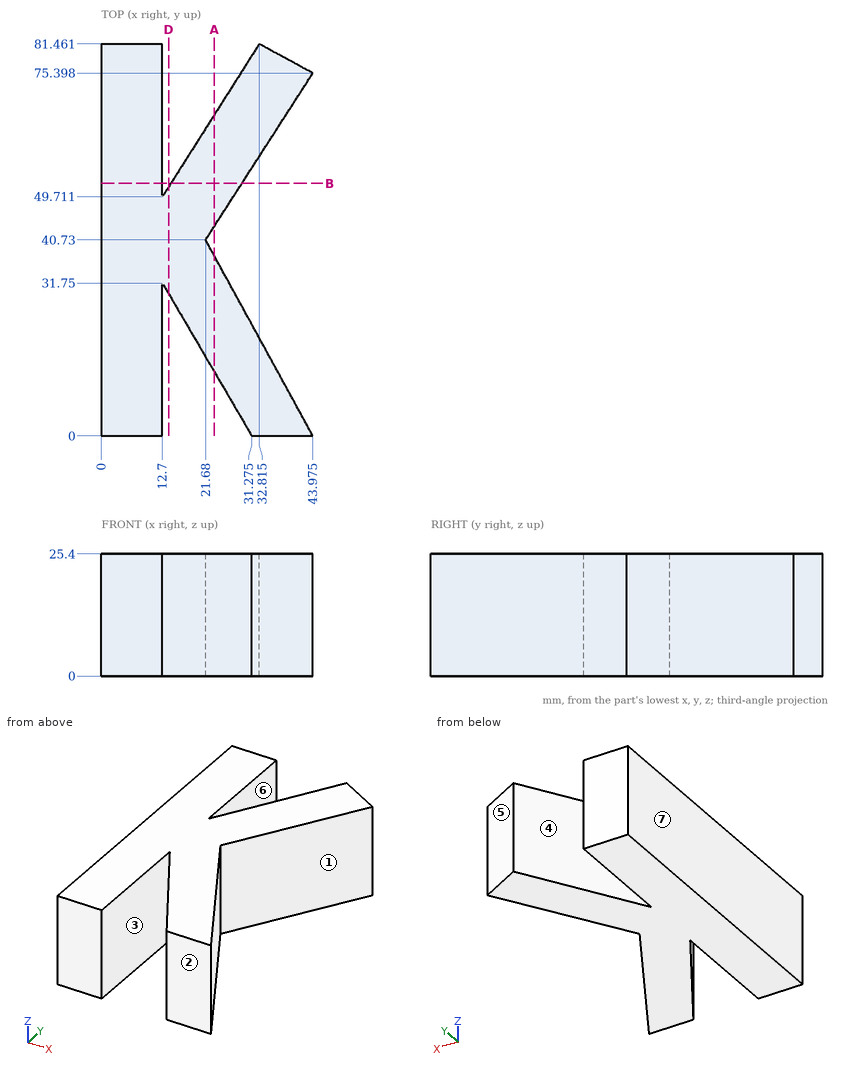
Can you work these out from the drawing? Everything is in mm from the part's minimum corner. A direction names the side the tool comes from. Coordinates: 2 decimals unless noted, no trailing zeros. Write each loop counter-clockwise with the first axis right and the second up, starting at its lowest first coordinate (ties: lowest second). Pieces come first, ordered by that corner, then holes. Notation, with made-up numbers: (-12, 89) -> (-5, 89) arc R34 cw to (-5, 124) -> close; hole circle Ø11 at (9.25, 35.25). An arc over 180 degrees is marked (long way). Return JSON: item names as keys, results as strings.
(1) I'm going to push flat-ended pins straight in: pin 1 (1 mm diameter, centred on y = 37.5, z = 8, fed in from -X); pin 2 (4 mm diameter, centred on x = 18.5, z = 3.5, fed in from -Y) (1 decimal); pin 3 (4 mm diameter, centred on y = 31.5, z = 12, fed in from +X); pin 4 (2 mm diameter, centred on x = 20, z = 8.5, fed in from +Y). Where does each tip first touch, or does it pass through?
Numbers:
{"pin 1": "stops at x = 0", "pin 2": "stops at y = 18.4", "pin 3": "stops at x = 27.83", "pin 4": "stops at y = 62.81"}
(2) Imagine slicing it at B-B, the plane y = 52.5. Please give me the cut outline in (x, z).
Numbers:
{"outline": "(0, 0) -> (12.7, 0) -> (12.7, 25.4) -> (0, 25.4) -> close; (14.47, 0) -> (29.25, 0) -> (29.25, 25.4) -> (14.47, 25.4) -> close"}
(3) Which directions (+Z, -Z, +X, -X, +Y, -Y) give clear straight access to the entire face, cutting with the end or side of a thin tool? Please do the marked faces 1, 2 and 3.
Numbers:
{"face 1": "+Z, -Z, +X", "face 2": "+Z, -Z, +X, -X, -Y", "face 3": "+Z, -Z, -Y"}
(4) I need wall thicknesses on L1, parallel to Y at x = 26.5, z = 3.75 (1 decimal); L2, parallel to Y at x = 30, z = 19.5 (1 decimal); L3, parallel to X at y = 16.5, z = 1.5 (1 decimal). Which ranges of each line are inside material? Lowest first, please.
Numbers:
{"L1": "y = 8.2 to 31.9, 48.2 to 71.5", "L2": "y = 2.2 to 25.5, 53.7 to 77", "L3": "x = 0 to 12.7, 21.6 to 34.9"}
(5) Imagine slicing it at D-D, the plane x = 14. Please give me the cut outline in (y, z).
Numbers:
{"outline": "(29.53, 0) -> (51.76, 0) -> (51.76, 25.4) -> (29.53, 25.4) -> close"}
(6) We'd pull the mould along X, two halves only. Please class the marked faces 4, 5, 6 and 7: +X half, -X half, draft (parallel to the pull), parting line (faces both ways), or undercut.
Numbers:
{"face 4": "undercut", "face 5": "+X half", "face 6": "undercut", "face 7": "-X half"}
(7) Imagine slicing it at A-A, the plane x = 23.5. Please give me the cut outline in (y, z) (1 decimal).
Numbers:
{"outline": "(13.3, 0) -> (37.4, 0) -> (37.4, 25.4) -> (13.3, 25.4) -> close; (43.6, 0) -> (66.8, 0) -> (66.8, 25.4) -> (43.6, 25.4) -> close"}
